Part print with two shaded views. Sizes in mm from the minimum x, y, z corner. A direction names the side the tool comes from. Coordinates: 2 decimals unless noted, no trailing zeros. Loops run counter-clockwise (first coordinate to the right, second up) from the corner with the lowest first, then second, coordinate; pieces in that order, holes last. Notation, with made-up numbers: M 3,-28.5 L 31,-28.5 A30 cw 31,-2.5 Z; hole C 34,-7 d4. An arc over 180 degrees is marked long. Write item = value, one per line. Start each with the question number.
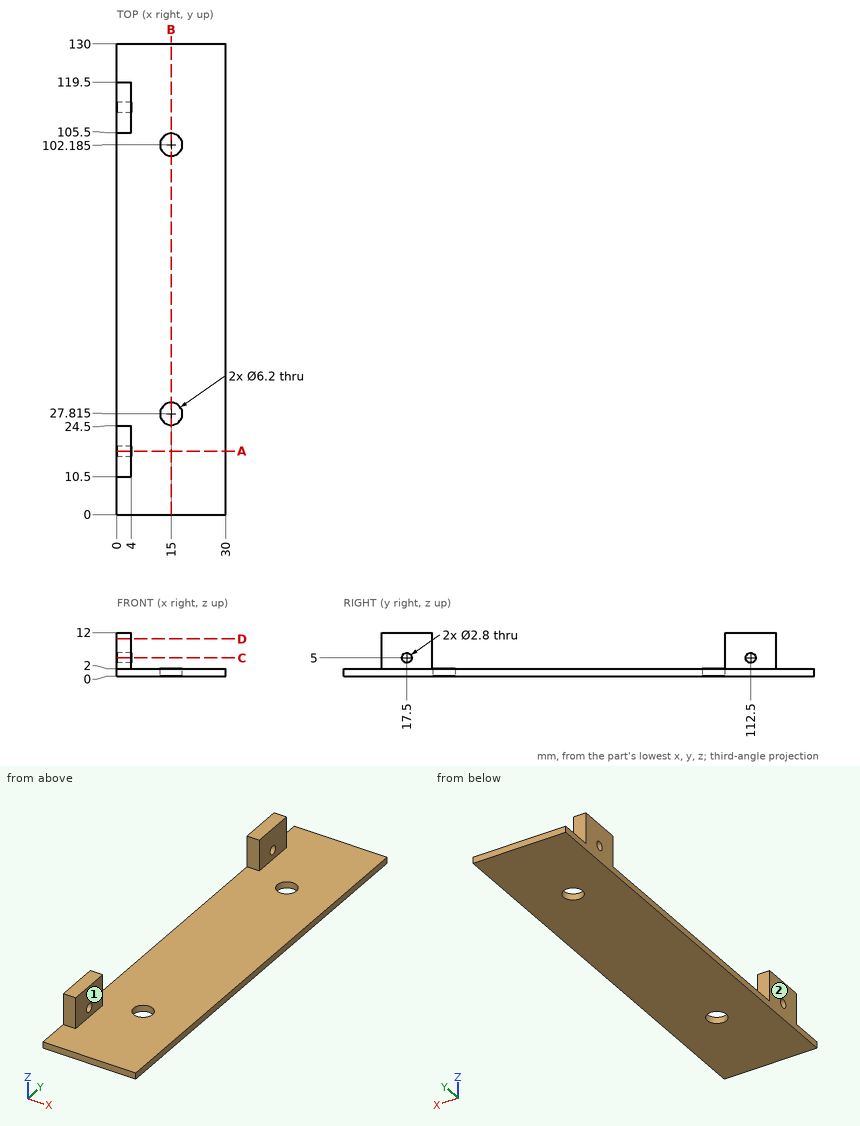
Item 1: Pin check, flat tips, straight feed: pin 1 Ø3 at (y, z) = (112.5, 9) entering from +X; pin 2 Ø4.5 at (x, z) = (2, 7) entering from -Y; pin 3 Ø1.2 at (x, z) = (3, 7.5) entering from +Y. Stop position of each tip, or through.
Item 2: Cut at B-B (x = 15). Give the cut face in (y, z) (1 decimal).
Item 3: Probe L1, parallel to Y at x = 15, z = 1.1 (1 decimal); L2, parallel to Y at x = 3.5, z = 5.5; L3, parallel to Z at x = 25.5, y = 110.5. List the from-to ranges inside material, lowest first.
Item 4: 3-axis set-ups, long thin cutter, end or side, ignore diameter. For the marked faces 1 and 2: which of +Z, -Z, +X, -X, +Y, -Y reach the whole face in a straight line?
Item 5: Cut at A-A (y = 17.5). Give the cut face in (x, z).
Item 6: Cut at D-D (z = 10.25). Give the cut face in (x, y).
Item 7: Cut at C-C (z = 5). Give the cut face in (x, y).
Reported:
q1.pin_1 = 4
q1.pin_2 = 10.5
q1.pin_3 = 119.5
q2.outline = M 0,0 L 24.7,0 L 24.7,2 L 0,2 Z; M 30.9,0 L 99.1,0 L 99.1,2 L 30.9,2 Z; M 105.3,0 L 130,0 L 130,2 L 105.3,2 Z
q3.L1 = 0 to 24.7, 30.9 to 99.1, 105.3 to 130
q3.L2 = 10.5 to 16.19, 18.81 to 24.5, 105.5 to 111.19, 113.81 to 119.5
q3.L3 = 0 to 2
q4.face_1 = +Z, +X, +Y, -Y
q4.face_2 = +Z, -Z, -X, +Y, -Y
q5.outline = M 0,0 L 30,0 L 30,2 L 4,2 L 4,3.6 L 0,3.6 Z; M 0,6.4 L 4,6.4 L 4,12 L 0,12 Z
q6.outline = M 0,10.5 L 4,10.5 L 4,24.5 L 0,24.5 Z; M 0,105.5 L 4,105.5 L 4,119.5 L 0,119.5 Z
q7.outline = M 0,10.5 L 4,10.5 L 4,16.1 L 0,16.1 Z; M 0,18.9 L 4,18.9 L 4,24.5 L 0,24.5 Z; M 0,105.5 L 4,105.5 L 4,111.1 L 0,111.1 Z; M 0,113.9 L 4,113.9 L 4,119.5 L 0,119.5 Z
